Autodesk Inventor part; units mm, degrees
ref_plane "YZ Plane" through (0, 0, 0) normal (1, 0, 0) x (0, 1, 0)
ref_plane "XZ Plane" through (0, 0, 0) normal (0, 1, 0) x (-1, 0, 0)
ref_plane "XY Plane" through (0, 0, 0) normal (0, 0, 1) x (1, 0, 0)
sketch "Sketch1" plane through (0, 0, 0) normal (0, 0, 1) x (1, 0, 0)
  line L0 (0, 0) -> (0, 80)
  line L1 (0, 0) -> (83, 0)
  line L2 (83, 16.7925) -> (83, 0)
  line L3 (0, 80) -> (83, 16.7925)
  dimension "d0" = 80
  dimension "d1" = 83
extrude "Extrusion1" add sketch "Sketch1" along normal blind 90
shell "Shell1" thickness 2 removed faces 2 at (27.6667, 0, 60) at (83, 5.5975, 30)
sketch "Sketch2" plane through (0, 0, 0) normal (-1, 0, 0) x (0, 0, 1)
  circle A0 centre (13.25, 32.7) radius 2.125
  circle A1 centre (13.25, 7.3) radius 2.125
  circle A2 centre (76.75, 32.7) radius 2.125
  line L0 (90, 80) -> (90, 0)
  line L1 (0, 80) -> (0, 0)
  circle A3 centre (76.75, 7.3) radius 2.125
  line L2 (0, 0) -> (90, 0)
  line L3 (0, 80) -> (90, 80)
  circle A4 centre (13.25, 58.1) radius 2.125
  circle A5 centre (76.75, 58.1) radius 2.125
  dimension "d5" = 4.25
  dimension "d6" = 4.25
  dimension "d7" = 4.25
  dimension "d8" = 63.5
  dimension "d10" = 13.25
  dimension "d11" = 25.4
  dimension "d12" = 4.25
  dimension "d13" = 63.5
  dimension "d14" = 7.3
  dimension "d15" = 7.3
  dimension "d28" = 13.25
  dimension "d36" = 4.25
  dimension "d37" = 4.25
  dimension "d38" = 25.4
  dimension "d39" = 25.4
  dimension "d40" = 21.9
  dimension "d41" = 21.9
  dimension "d42" = 13.25
extrude "Extrusion2" cut sketch "Sketch2" against normal blind 2 contours A0 | A1 | A2 | A3 | A4 | A5
sketch "Sketch3" plane through (0, 0, 90) normal (0, 0, 1) x (1, 0, 0)
  circle A0 centre (78.5, 8.5093) radius 2.5
  line L0 (83, 0) -> (83, 16.7925)
  line L1 (83, 16.7925) -> (0, 80)
  point P0 (0, 0)
  point P1 (83, 8.3963)
  dimension "d19" = 5
  dimension "d20" = 4.5
  dimension "d21" = 9.3163
extrude "Extrusion3" cut sketch "Sketch3" against normal blind 2
sketch "Sketch4" plane through (0, 0, 0) normal (0, 0, -1) x (-1, 0, 0)
  circle A0 centre (-78.5, 8.5093) radius 2.5
  circle A1 centre (-78.5, 8.5093) radius 2.5
  point P0 (0, 0)
  dimension "d24" = 5
extrude "Extrusion4" cut sketch "Sketch4" against normal blind 2
sketch "Sketch7" plane through (2, 0, 2) normal (0, 0, 1) x (1, 0, 0)
  line L0 (81, 0) -> (0, 0)
  line L1 (0, 75.963) -> (0, 0)
  line L2 (0, 0) -> (0, 75.963)
  line L3 (81, 14.2786) -> (81, 0)
  line L4 (0, 75.963) -> (81, 14.2786)
  line L5 (81, 14.2786) -> (81, 0)
  line L6 (81, 0) -> (0, 0)
  point P0 (-2, 0)
extrude "Extrusion7" cut sketch "Sketch7" against normal blind 2
sketch "Sketch8" plane through (83, 0, 88) normal (0, 0, -1) x (-1, 0, 0)
  line L0 (0, 0) -> (0, 14.2786)
  line L1 (0, 0) -> (0, 16.7925)
  line L2 (0, 14.2786) -> (0, 0)
  line L3 (81, 75.963) -> (81, 0)
  line L4 (0, 0) -> (81, 0)
  line L5 (81, 0) -> (81, 75.963)
  line L6 (81, 75.963) -> (0, 14.2786)
  line L7 (0, 16.7925) -> (83, 80)
  point P0 (83, 0)
extrude "Extrusion8" cut sketch "Sketch8" against normal blind 2
properties part number "P1D1_2Ramp"
Model file for the job. Use its own axes, mm. A direction names the side the tool comes from. Give positions to 0.01 mm unless a question says otherwise; leave off trailing zeros. Loops run counter-clockwise (first coordinate to the right, second up) from the corner with the lowest first, then second, coordinate; pieces in that order, holes last.
1) Saw through at B-B (y = 32.7). Write the cut outline in (x, z) (3 decimals), plus the area to 3 significant figures.
2) Pull direction Z, two halves, no side cores. Call faces 4 (the flat face through (41.933, 45.553, 1.014)), 5 (the flat face through (26, 58, 0)), 6 (the cylindrical face through (0.99, 31.41, 75.06)), 7 (the cylindrical face through (0.986, 30.626, 12.789)): +Z half, -Z half, draft (parallel to the pull), parting line (faces both ways), or undercut.
3) Saw through at D-D (z = 51). Write the cut outline in (x, y).
4) Saw through at C-C (y = 7.3). Write the cut outline in (x, z) (3 decimals), plus the area to 3 significant figures.
5) Tool access for faces 1 (the cylindrical face through (0.99, 56.81, 75.06)), 2 (the flat face through (26, 58, 90)), 3 (the flat face through (41.933, 45.553, 88.986)): list every direction of +Z, -Z, +X, -X, +Y, -Y with a clear straight run to the whole face (end or side of a thin tool).
6) Flat gauge pins, fed straight in: pin 1 Ø10 at (y, z) = (57.5, 78.5) entering from +X; pin 2 Ø7 at (y, z) = (58.1, 76.75) entering from +X; pin 3 Ø6 at (y, z) = (70, 16.5) entering from +X. Where does each tip first touch, or does it go through?
7) Saw through at A-A (z = 13.25). Write the cut outline in (x, y) (1 decimal).
8) Wall check: line 1 (Y direction, x = 1.5, z = 13.25) (3 decimals); line 2 (Z direction, x = 1, y = 58); line 3 (Y direction, x = 0.9, z = 13.25) (3 decimals). Give the ranges that are in metal, low to high.
Answer block:
1. outline: (0, 0) - (2, 0) - (2, 11.125) - (0, 11.125) - close; (0, 15.375) - (2, 15.375) - (2, 74.625) - (0, 74.625) - close; (0, 78.875) - (2, 78.875) - (2, 90) - (0, 90) - close; (58.81, 0) - (62.111, 0) - (62.111, 90) - (58.81, 90) - close
1. area: 460 mm2
2. face 4: draft
2. face 5: -Z half
2. face 6: undercut
2. face 7: undercut
3. outline: (0, 0) - (2, 0) - (2, 75.96) - (83, 14.28) - (83, 16.79) - (0, 80) - close
4. outline: (0, 0) - (2, 0) - (2, 11.125) - (0, 11.125) - close; (0, 15.375) - (2, 15.375) - (2, 74.625) - (0, 74.625) - close; (0, 78.875) - (2, 78.875) - (2, 90) - (0, 90) - close
4. area: 163 mm2
5. face 1: -X
5. face 2: +Z, +X, -X, +Y, -Y
5. face 3: +Z, -Z, -Y
6. pin 1: stops at x = 36.11
6. pin 2: stops at x = 33.35
6. pin 3: stops at x = 17.07
7. outline: (0, 0) - (2, 0) - (2, 5.2) - (0, 5.2) - close; (0, 9.4) - (2, 9.4) - (2, 30.6) - (0, 30.6) - close; (0, 34.8) - (2, 34.8) - (2, 56) - (0, 56) - close; (0, 60.2) - (2, 60.2) - (2, 76) - (83, 14.3) - (83, 16.8) - (0, 80) - close
8. line 1: y = 0 to 5.175, 9.425 to 30.575, 34.825 to 55.975, 60.225 to 78.858
8. line 2: z = 0 to 11.13, 15.37 to 74.63, 78.87 to 90
8. line 3: y = 0 to 5.175, 9.425 to 30.575, 34.825 to 55.975, 60.225 to 79.315
